Could you check a few things on this model? Use its own coordinates, in mm. A direction names the side the tool comes from. Coordinates: 2 decimals unless noted, no trailing zeros. Loops run counter-clockwise (first coordinate to the right, second up) from the corner with the lowest first, then second, coordinate; pieces in that order, holes last.
1) Imagine slicing it at A-A on z = 0. Please give me the cut outline in (x, y), plus the area to 3 significant figures.
2) For faces 4 (the face through (0.748, 5.198, -0.976)), 5 (the face through (-2, 10.5, 0)), 6 (the face through (0.748, -5.198, 0.976)), which set-ups out of +Z, -Z, +X, -X, +Y, -Y let a thin tool reach every point of the face, with its end or its side?
3) Will these pins go through, and if not, where does the flat tip stop? P1, Ø1.5, axis at x = 2, y = -1.5, coming from the +Z side; P2, Ø1.5, axis at x = 0, z = 0, coming from the -Y side; P3, Ø2, axis at x = 0, z = 0, coming from the +Y side.
4) If I drill on line 1 along Z through (x, y) = (0, 7.25); line 2 along Y through (x, z) = (0.6, 0.5); line 3 along X through (y, z) = (-2.5, 1.05), over which ranges is the centre line in solid material (lowest first)?
5) Imagine slicing it at B-B on y = -6.5. Please give me the cut outline in (x, z).
6) Imagine slicing it at C-C on x = 0. Please give me the cut outline in (y, z), plus the area to 3 significant figures.
7) Thinking about a two-plate mould opening in Z: for faces 1 (the face through (3, 0, 0)), 2 (the face through (0, 0.5, 0)), 3 (the face through (-2, -10.5, 0)), which applies, released by +Z, released by -Z, zero draft, split by the parting line, or undercut?
Autodesk Inventor part; units mm, degrees
ref_plane "YZ Plane" through (0, 0, 0) normal (1, 0, 0) x (0, 1, 0)
ref_plane "XZ Plane" through (0, 0, 0) normal (0, 1, 0) x (-1, 0, 0)
ref_plane "XY Plane" through (0, 0, 0) normal (0, 0, 1) x (1, 0, 0)
sketch "スケッチ1" plane through (0, 0, 0) normal (0, 1, 0) x (-1, 0, 0)
  circle A0 centre (0, 0) radius 3
  dimension "d0" = 6
extrude "押し出し1" add sketch "スケッチ1" along normal mid plane 21
sketch "スケッチ2" plane through (0, 10.5, 0) normal (0, 1, 0) x (1, 0, 0)
  point P0 (0, 0)
  point P1 (0, 0)
hole "穴1" at (0, 10.5, 0) direction (0, -1, 0) diameter 2.459 depth 10 countersink diameter 3.4 countersink angle 90
sketch "スケッチ3" plane through (0, -10.5, 0) normal (0, -1, 0) x (1, 0, 0)
  point P0 (0, 0)
  point P1 (0, 0)
hole "穴2" at (0, -10.5, 0) direction (0, 1, 0) diameter 2.459 depth 10 countersink diameter 3.4 countersink angle 90
chamfer "面取り1" distance 0.25 angle 45 2 edges at (3, -10.5, 0) (3, 10.5, 0)
properties part number "Spacer_M3D6L60" material "アルミニウム 6061"
Filled in:
1. outline: (-3, -10.25) - (-2.75, -10.5) - (-1.7, -10.5) - (-1.23, -10.03) - (-1.23, -0.5) - (1.23, -0.5) - (1.23, -10.03) - (1.7, -10.5) - (2.75, -10.5) - (3, -10.25) - (3, 10.25) - (2.75, 10.5) - (1.7, 10.5) - (1.23, 10.03) - (1.23, 0.5) - (-1.23, 0.5) - (-1.23, 10.03) - (-1.7, 10.5) - (-2.75, 10.5) - (-3, 10.25) - close
1. area: 76.3 mm2
2. face 4: +Y
2. face 5: +Z, -Z, +X, -X, +Y
2. face 6: -Y
3. P1: stops at z = 2.73
3. P2: stops at y = -0.5
3. P3: stops at y = 0.5
4. line 1: z = -3 to -1.23, 1.23 to 3
4. line 2: y = -0.5 to 0.5
4. line 3: x = -2.81 to -0.64, 0.64 to 2.81
5. outline: circle Ø6 at (0, 0); hole circle Ø2.46 at (0, 0)
6. outline: (-10.5, -2.75) - (-10.25, -3) - (10.25, -3) - (10.5, -2.75) - (10.5, -1.7) - (10.03, -1.23) - (0.5, -1.23) - (0.5, 1.23) - (10.03, 1.23) - (10.5, 1.7) - (10.5, 2.75) - (10.25, 3) - (-10.25, 3) - (-10.5, 2.75) - (-10.5, 1.7) - (-10.03, 1.23) - (-0.5, 1.23) - (-0.5, -1.23) - (-10.03, -1.23) - (-10.5, -1.7) - close
6. area: 76.3 mm2
7. face 1: split by the parting line
7. face 2: undercut
7. face 3: zero draft
